Part model, mm, in its own coordinate system. A direction names the side the tool comes from. Coordinates: 2 decimals unless noted, no trailing zeros. Write each loop counter-clockwise with the first axis right and the second up, starting at its lowest first coordinate (ties: lowest second). Pieces come first, ordered by that corner, then holes. Notation, with made-up numbers: (-5, 4.25) - (19, 4.25) arc R19 ccw to (19, 36.25) - close; hole circle Ø7 at (84, -35.75). An arc over 180 degrees is marked (long way). Use a Markdown table: item, result.
```python
from build123d import *

# Parameters (mm, degrees)
SKETCH002_W      = 20
SKETCH002_H      = 20
SKETCH002_W_2    = 22
SKETCH002_H_2    = 22
EXTRUDE_DEPTH    = 1
SKETCH001_R      = 2.75
EXTRUDE002_DEPTH = 5
SKETCH_W         = 169
SKETCH_H         = 169
EXTRUDE001_DEPTH = 2


with BuildPart() as cutouts:
    # Sketch002 → Extrude (new body, symmetric)
    with BuildSketch(Plane.XY.offset(2)):
        with Locations((0, -65)):
            Rectangle(SKETCH002_W, SKETCH002_H)
        with Locations((0, 70)):
            Rectangle(SKETCH002_W_2, SKETCH002_H_2)
    extrude(amount=EXTRUDE_DEPTH, both=True)


with BuildPart() as mountholes:
    # Sketch001 → Extrude002 (new body, symmetric)
    with BuildSketch(Plane.XY.offset(2)):
        with Locations((-75, -75)):
            Circle(SKETCH001_R)
        with Locations((75, -75)):
            Circle(SKETCH001_R)
        with Locations((75, 75)):
            Circle(SKETCH001_R)
        with Locations((-75, 75)):
            Circle(SKETCH001_R)
    extrude(amount=EXTRUDE002_DEPTH, both=True)


with BuildPart() as cut001:
    # Sketch → Extrude001 (new body)
    with BuildSketch(Plane.XY):
        Rectangle(SKETCH_W, SKETCH_H)
    extrude(amount=EXTRUDE001_DEPTH)

    # Cut: cut MountHoles
    add(mountholes.part, mode=Mode.SUBTRACT)

    # Cut001: cut Cutouts
    add(cutouts.part, mode=Mode.SUBTRACT)


solid = cut001.part
```
Item 1: Band-saw the part on C-C, the plane y = 75. Give the cut face in (x, z), then the cut area to 3 significant figures.
From the geometry:
| item | result |
|---|---|
| outline | (-84.5, 0) - (-77.75, 0) - (-77.75, 2) - (-84.5, 2) - close; (-72.25, 0) - (72.25, 0) - (72.25, 2) - (11, 2) - (11, 1) - (-11, 1) - (-11, 2) - (-72.25, 2) - close; (77.75, 0) - (84.5, 0) - (84.5, 2) - (77.75, 2) - close |
| area | 294 mm^2 |
Item 2: Two-plate mould, pull along Y, no slides. Class faces 3 (the face through (72.973, -73.141, 1.014)), 4 (the face through (-1, 1, 2)): pulls with the +Y half, pulls with the -Y half, needs draft (parallel to the pull), parting line crosses it, or undercut.
From the geometry:
| item | result |
|---|---|
| face 3 | undercut |
| face 4 | needs draft |
Item 3: Drop a flat-ended pin along its axis: P1, Ø6.5, axis at x = 3, y = 72.5, coming from the +Z side. Give the stop position or say it passes through.
From the geometry:
| item | result |
|---|---|
| P1 | z = 1 |
Item 4: Band-saw the part on B-B, the plane z = 1.45. Give the cut face in (x, y), then the cut area to 3 significant figures.
From the geometry:
| item | result |
|---|---|
| outline | (-84.5, -84.5) - (84.5, -84.5) - (84.5, 84.5) - (-84.5, 84.5) - close; hole circle Ø5.5 at (-75, -75); hole circle Ø5.5 at (-75, 75); hole (-11, 59) - (11, 59) - (11, 81) - (-11, 81) - close; hole (-10, -75) - (10, -75) - (10, -55) - (-10, -55) - close; hole circle Ø5.5 at (75, -75); hole circle Ø5.5 at (75, 75) |
| area | 27,600 mm^2 |
Item 5: Band-saw the part on A-A, the plane x = -75. Give the cut face in (y, z), then the cut area to 3 significant figures.
From the geometry:
| item | result |
|---|---|
| outline | (-84.5, 0) - (-77.75, 0) - (-77.75, 2) - (-84.5, 2) - close; (-72.25, 0) - (72.25, 0) - (72.25, 2) - (-72.25, 2) - close; (77.75, 0) - (84.5, 0) - (84.5, 2) - (77.75, 2) - close |
| area | 316 mm^2 |
Item 6: Which spindle directions (+Z, -Z, +X, -X, +Y, -Y) get a long thin tool onto all of the face, cutting with end or side? Do faces 1 (the face through (72.253, 75.121, 1.014)), 2 (the face through (0, 70, 1)). Say none if no direction does.
From the geometry:
| item | result |
|---|---|
| face 1 | +Z, -Z |
| face 2 | +Z |
Item 7: Drill centre lines: probe 1 along Y at (x, z) = (75, 0.9); probe 2 along Y at (x, z) = (1.5, 1.1); probe 3 along X at (y, z) = (-60.5, 1.45). Where is each one in solid material? Low to high.
From the geometry:
| item | result |
|---|---|
| probe 1 | -84.5 to -77.75, -72.25 to 72.25, 77.75 to 84.5 |
| probe 2 | -84.5 to -75, -55 to 59, 81 to 84.5 |
| probe 3 | -84.5 to -10, 10 to 84.5 |
